For this review, use the dimensioned drawing (mm, ordinates from the lowest corner) and the shaded views. Give positions to 0.01 mm unless a question says otherwise; leave off trailing zeros. Order: outer loops, then holes, each group sorted by start corner. A loop starts at its lowest first (then second) coordinate and runs counter-clockwise, first axis right, second up. Notation, with made-up numbers: (-20.5, -21.75) - (-13.5, -21.75) arc R30 cw to (-13.5, 9.25) - close; hole circle Ø11 at (48, -31.75). An arc over 180 degrees is marked (long way). Use a Markdown table: item, result. Add a question column.
1) We need section A-A on y = 2.75. Write out the cut boundary in (x, z).
2) Clearance check with a flat-ended pin moving along its axis: P1, Ø2, axis at x = 17, z = 17, coming from the -Y side. State where the tip first meets the part, or that it passes through.
3) We need section B-B on x = 2.25. Write out the cut boundary in (y, z).
4) We need section C-C on z = 18.75. Write out the cut boundary in (x, y).
5) Mouldability with a two-part tool opening along Z and no side actions: class the marked faces 1, 2 and 3 as released by +Z, released by -Z, zero draft, split by the parting line, or undercut.
6) Wall thickness on L1, parallel to X at y = 2.45, z = 17; L2, parallel to Z at x = 17, y = 4.1; L3, parallel to X at y = 4.2, z = 18: over which ranges is each line inside the solid? List them lowest first.
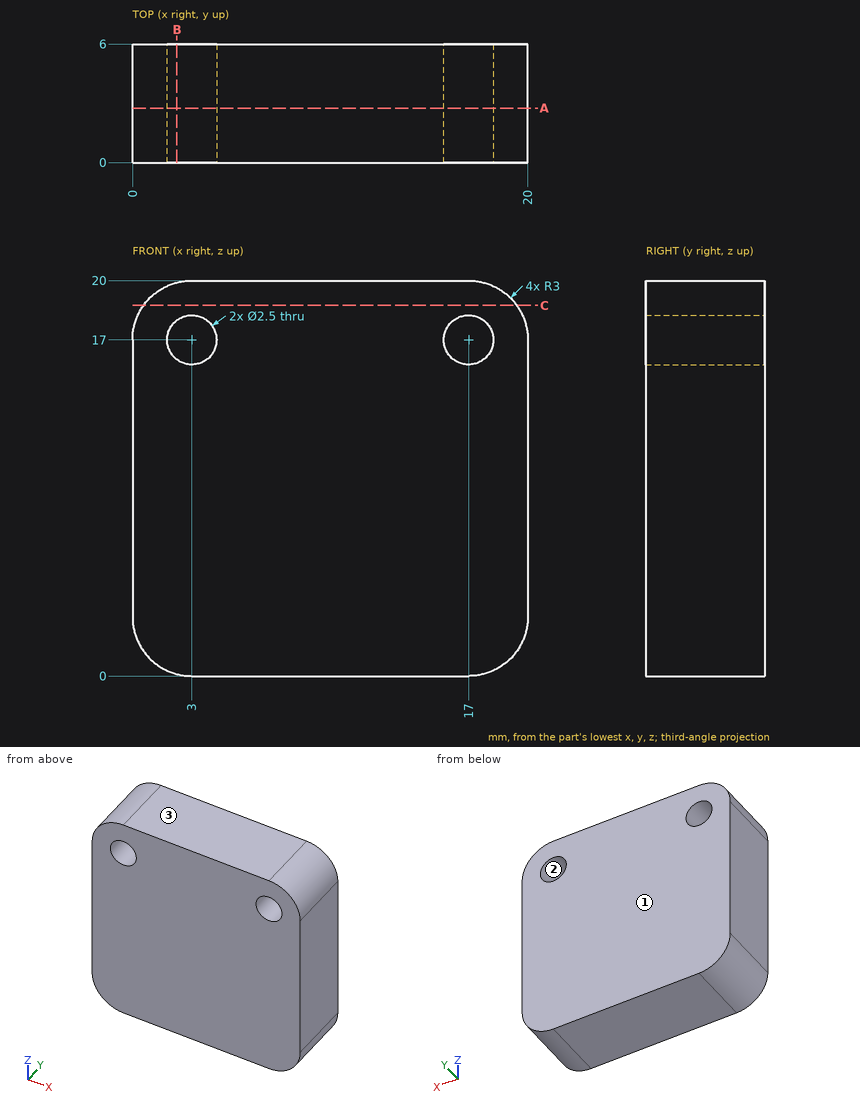
Checked values:
| question | item | result |
|---|---|---|
| 1 | outline | (0, 3) arc R3 ccw to (3, 0) - (17, 0) arc R3 ccw to (20, 3) - (20, 17) arc R3 ccw to (17, 20) - (3, 20) arc R3 ccw to (0, 17) - close; hole circle Ø2.5 at (3, 17); hole circle Ø2.5 at (17, 17) |
| 2 | P1 | through |
| 3 | outline | (0, 0.1) - (6, 0.1) - (6, 16) - (0, 16) - close; (0, 18) - (6, 18) - (6, 19.9) - (0, 19.9) - close |
| 4 | outline | (0.56, 0) - (19.44, 0) - (19.44, 6) - (0.56, 6) - close |
| 5 | face 1 | zero draft |
| 5 | face 2 | undercut |
| 5 | face 3 | released by +Z |
| 6 | L1 | 0 to 1.75, 4.25 to 15.75, 18.25 to 20 |
| 6 | L2 | 0 to 15.75, 18.25 to 20 |
| 6 | L3 | 0.17 to 2.25, 3.75 to 16.25, 17.75 to 19.83 |
